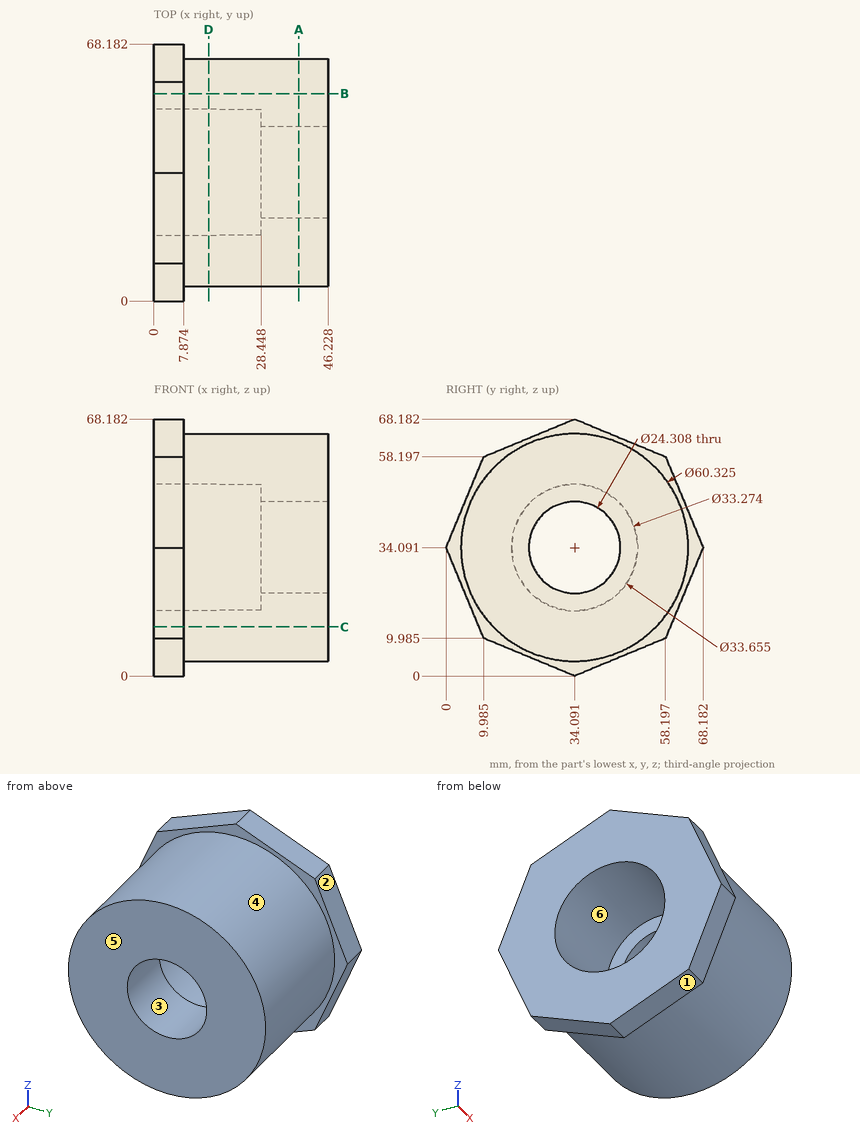
Answer from the drawing. Dimensions are ordinates in mm from the lowest x, y and z of the part. A direction names the side the tool comes from. Coordinates: 2 decimals unless noted, no trailing zeros. Loops run counter-clockwise (first coordinate to the right, second up) from the corner with the lowest first, then second, coordinate; pieces in that order, holes last. Notation, with made-up numbers: (75, -1.5) -> (133, -1.5) arc R23 cw to (133, 36.5) -> close; hole circle Ø7 at (15.5, 52.25). An arc over 180 degrees is marked (long way). Return JSON: item names as keys, results as strings.
Item 1: Find section B-B (y = 55). Determine the outline of the cut face in (x, z), plus the area to 3 significant figures.
Answers:
{"outline": "(0, 8.66) -> (7.87, 8.66) -> (7.87, 12.35) -> (46.23, 12.35) -> (46.23, 55.83) -> (7.87, 55.83) -> (7.87, 59.52) -> (0, 59.52) -> close", "area": "2,070 mm2"}
Item 2: Find section D-D (x = 14.5). Determine the outline of the cut face in (y, z) (1 decimal), plus the area to 3 significant figures.
Answers:
{"outline": "circle Ø60.3 at (34.1, 34.1); hole circle Ø33.5 at (34.1, 34.1)", "area": "1,980 mm2"}
Item 3: Find the intervals of material crossed by probe 1 along Z at (x, y) = (44, 33.5); probe 2 along Z at (x, y) = (39, 30) (1 decimal); probe 3 along Y at (x, z) = (10.5, 23), in increasing order.
Answers:
{"probe 1": "z = 3.93 to 21.95, 46.23 to 64.25", "probe 2": "z = 4.2 to 22.6, 45.5 to 64", "probe 3": "y = 6.04 to 21.53, 46.65 to 62.14"}
Item 4: Flat-ended cylindrical pins translate along their axes: P1, Ø10, axis at y = 55.5, z = 60.5, coming from the +X side; P2, Ø2, axis at x = 7, y = 51.5, coming from the +Z side (1 decimal); P3, Ø5, axis at x = 16.5, y = 33.5, coming from the -Z side; P4, Ø22, axis at y = 34.09, z = 34.09, coming from the -X side. Find the tip coordinate at first contact, or state that the pin passes through.
Answers:
{"P1": "stops at x = 46.23", "P2": "stops at z = 61.4", "P3": "stops at z = 3.93", "P4": "passes through"}
Item 5: For the marked faces 4, 5 and 6, determine the directions among +Z, -Z, +X, -X, +Y, -Y from which every point of the face is accessible in a straight line to the end or side of a thin tool.
Answers:
{"face 4": "+X", "face 5": "+Z, -Z, +X, +Y, -Y", "face 6": "-X"}
Item 6: For a pull along Z with two mould halves and no side action, classify the marked faces 1, 2 and 3 as +Z half, -Z half, draft (parallel to the pull), parting line (faces both ways), or undercut.
Answers:
{"face 1": "-Z half", "face 2": "+Z half", "face 3": "undercut"}
Item 7: Find section A-A (x = 38.5). Determine the outline of the cut face in (y, z) (1 decimal).
Answers:
{"outline": "circle Ø60.3 at (34.1, 34.1); hole circle Ø24.3 at (34.1, 34.1)"}
Item 8: Find section C-C (z = 13). Determine the outline of the cut face in (x, y).
Answers:
{"outline": "(0, 8.74) -> (7.87, 8.74) -> (7.87, 12.53) -> (46.23, 12.53) -> (46.23, 55.65) -> (7.87, 55.65) -> (7.87, 59.45) -> (0, 59.45) -> close"}
